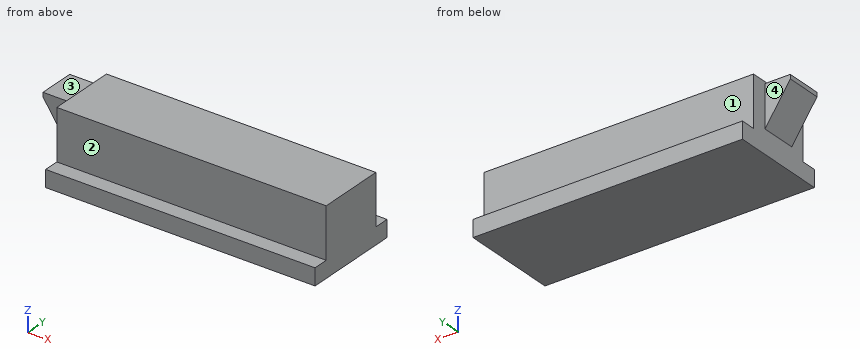
from build123d import *

# Parameters (mm, degrees)
F1_DEPTH = 4
F2_DEPTH = 2.15
F0_W     = 32
F0_H     = 2
F3_DEPTH = 5.8


with BuildPart() as f1:
    # F0 (on Front) → F1 (new body, symmetric)
    with BuildSketch(Plane.XZ):
        Polygon((-13.8378396917, 2.8), (-13.8378396917, 2), (18.1621603083, 2), (18.1621603083, 8), (-13.8378396917, 8), (-13.8378396917, 7.8), align=None)
    extrude(amount=F1_DEPTH, both=True)

    # F0 (on Front) → F2 (join, symmetric)
    with BuildSketch(Plane.XZ):
        Polygon((-16.8378396917, 7.3), (-13.8378396917, 2.8), (-13.8378396917, 7.8), (-16.8378396917, 7.8), align=None)
    extrude(amount=F2_DEPTH, both=True)

    # F0 (on Front) → F3 (join, symmetric)
    with BuildSketch(Plane.XZ):
        with Locations((2.1621603083, 1)):
            Rectangle(F0_W, F0_H)
    extrude(amount=F3_DEPTH, both=True)


solid = f1.part
Work out the finished part from the listing and answer in its coordinate system (mm). Face numbers are marked on the shaded views. A direction names the side the tool comes from. Give positions to 0.01 mm unless a question says otherwise; leave off trailing zeros. Write each loop counter-clockwise with the first axis right and the second up, starting at its lowest first coordinate (ties: lowest second). Pieces come first, ordered by that corner, then holes. Notation, with made-up numbers: (28.5, 50.25) - (36.5, 50.25) arc R12 ccw to (36.5, 58.25) - close; hole circle Ø5 at (-25.75, 48.5). An arc over 180 degrees is marked (long way). One line per item, written item: value. Start each with the question number.
1. Given pin 1 (0.9 mm diameter, centred on x = -14.5, y = 1, fed in from +Z); pin 2 (4 mm diameter, centred on y = -2, z = 4.5, fed in from -X); pin 3 (3 mm diameter, centred on y = 4, z = 1.5, fed in from -X), each flat-ended and moving along its own axis, determine where each tip first touches the part or whether it passes through.
2. Consider probe 1 along Z at (x, y) = (-6, 4.5); probe 2 along Y at (x, z) = (10.5, 6.5); probe 3 along X at (y, z) = (2.5, 2.75). Determine where each line is inside the solid, lowest interval first.
3. Find section B-B (y = 0.25). Write down the section's boundary in (x, z).
4. Find section C-C (z = 0.75). Write down the section's boundary in (x, y).
5. Find section A-A (x = 10). Write down the section's boundary in (y, z), then the cut area to 3 significant figures.
6. Find section D-D (y = 2.5). Write down the section's boundary in (x, z).
7. For the marked faces 1, 2, 3 and 4, determine the directions among +Z, -Z, +X, -X, +Y, -Y from which every point of the face is accessible in a straight line to the end or side of a thin tool.
Geometry results:
1. pin 1: z = 7.8
1. pin 2: x = -16.3
1. pin 3: x = -13.84
2. probe 1: 0 to 2
2. probe 2: -4 to 4
2. probe 3: -13.84 to 18.16
3. outline: (-16.84, 7.3) - (-13.84, 2.8) - (-13.84, 0) - (18.16, 0) - (18.16, 8) - (-13.84, 8) - (-13.84, 7.8) - (-16.84, 7.8) - close
4. outline: (-13.84, -5.8) - (18.16, -5.8) - (18.16, 5.8) - (-13.84, 5.8) - close
5. outline: (-5.8, 0) - (5.8, 0) - (5.8, 2) - (4, 2) - (4, 8) - (-4, 8) - (-4, 2) - (-5.8, 2) - close
5. area: 71.2 mm2
6. outline: (-13.84, 0) - (18.16, 0) - (18.16, 8) - (-13.84, 8) - close
7. face 1: +Z, +X, -X, +Y
7. face 2: +Z, +X, -X, -Y
7. face 3: +Z, -X, +Y, -Y
7. face 4: +Z, -Z, -X, +Y
